Geometry: final body of the model. Coordinates: model frame, mm. A direction names the side the tool comes from. Give positions to 0.01 mm unless a question says otherwise; leave off trailing zeros. Order: outer loops, then holes, each group sorted by start corner. A loop starts at its lowest first (then second) coordinate and runs counter-clockwise, first axis right, second up. Notation, with made-up numbers: (-31.5, -35.75) - (-10.5, -35.75) arc R22 ccw to (-10.5, -20.75) - close; hole circle Ø8 at (59, 70). An arc over 180 degrees is marked (long way). One line per item, written item: value.
```python
from build123d import *

# Parameters (mm, degrees)
F0_W     = 72.9460567236
F0_H     = 61.1247569323
F1_DEPTH = 38.1
F2_R     = 18.9050418051
F3_DEPTH = 50.8
F4_R     = 24.4111270382
F4_R_2   = 18.9050418051
F5_DEPTH = 25.4


with BuildPart() as f1:
    # F0 (on Front) → F1 (new body)
    with BuildSketch(Plane.XZ):
        Rectangle(F0_W, F0_H)
    extrude(amount=F1_DEPTH)

    # F2 (on face) → F3 (cut)
    with BuildSketch(Plane.XZ.offset(38.1)):
        Circle(F2_R)
    extrude(amount=-F3_DEPTH, mode=Mode.SUBTRACT)

    # F4 (on face) → F5 (join)
    with BuildSketch(Plane.XZ.offset(38.1)):
        Circle(F4_R)
        Circle(F4_R_2, mode=Mode.SUBTRACT)
    extrude(amount=F5_DEPTH)


solid = f1.part
```
1) First-contact query: pin 1 (5 mm diameter, centred on x = -18, z = -14.5, fed in from +Y); pin 2 (5 mm diameter, centred on x = 1, y = -49, fed in from -Z); pin 3 (10 mm diameter, centred on x = 25, y = -44.5, fed in from +Z). Flat tips, straight axial feed; report the tip coordinate or a pass-through.
Answers below:
pin 1: y = 0
pin 2: z = -24.41
pin 3: z = 14
2) Set-up query: faces 1 (the face through (-5.29, -50.62, -23.83)), 2 (the face through (-1, -19, 30.562)). Return all of +Z, -Z, +X, -X, +Y, -Y with unobstructed straight access to the full face (end or side cutting, diameter ignored); none if empty.
Answers below:
face 1: -Y
face 2: +Z, +X, -X, +Y, -Y
3) Material intervals for line 1 along Z through (x, y) = (0, -44); line 2 along X through (y, z) = (-30.5, -14); line 3 along X through (y, z) = (-46.5, 11), sorted ascending.
Answers below:
line 1: -24.41 to -18.91, 18.91 to 24.41
line 2: -36.47 to -12.7, 12.7 to 36.47
line 3: -21.79 to -15.38, 15.38 to 21.79
4) Section C-C, the plane y = -9.5. Return loops of the section in (x, z).
Answers below:
outline: (-36.47, -30.56) - (36.47, -30.56) - (36.47, 30.56) - (-36.47, 30.56) - close; hole circle Ø37.81 at (0, 0)
5) Section B-B, the plane x = 0. Return loops of the section in (y, z), then the cut area to 3 significant figures.
Answers below:
outline: (-63.5, -24.41) - (-38.1, -24.41) - (-38.1, -30.56) - (0, -30.56) - (0, -18.91) - (-63.5, -18.91) - close; (-63.5, 18.91) - (0, 18.91) - (0, 30.56) - (-38.1, 30.56) - (-38.1, 24.41) - (-63.5, 24.41) - close
area: 1,170 mm^2
6) Section A-A, the plane z = 0. Return loops of the section in (x, y).
Answers below:
outline: (-36.47, -38.1) - (-24.41, -38.1) - (-24.41, -63.5) - (-18.91, -63.5) - (-18.91, 0) - (-36.47, 0) - close; (18.91, -63.5) - (24.41, -63.5) - (24.41, -38.1) - (36.47, -38.1) - (36.47, 0) - (18.91, 0) - close
7) Section D-D, the plane x = -30. Return loops of the section in (y, z).
Answers below:
outline: (-38.1, -30.56) - (0, -30.56) - (0, 30.56) - (-38.1, 30.56) - close
